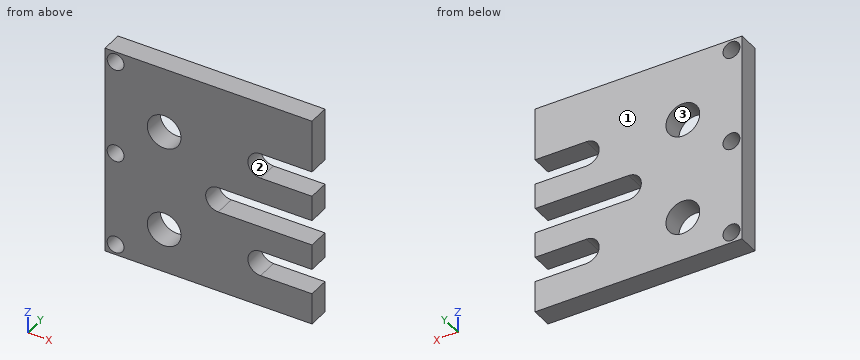
from build123d import *

# Parameters (mm, degrees)
F0_R     = 2
F0_R_2   = 4
F1_DEPTH = 5


with BuildPart() as f1:
    # F0 (on Front) → F1 (new body)
    with BuildSketch(Plane.XZ):
        with BuildLine():
            Line((-9.071991, 28.153977), (-9.071683, 40.657913))
            Line((-9.071683, 40.657913), (-58.072915, 40.657913))
            Line((-58.072915, 40.657913), (-58.072915, -9.342087))
            Line((-58.072915, -9.342087), (-9.072915, -9.342087))
            Line((-9.072915, -9.342087), (-9.072732, -1.896336))
            Line((-9.072732, -1.896336), (-21.245276, -1.896336))
            ThreePointArc((-21.245276, -1.896336), (-24.245276, 1.103664), (-21.245276, 4.103664))
            Line((-21.245276, 4.103664), (-9.082483, 4.103664))
            Line((-9.082483, 4.103664), (-9.072584, 4.103664))
            Line((-9.072584, 4.103664), (-9.072436, 10.135129))
            Line((-9.072436, 10.135129), (-31.243636, 10.135129))
            ThreePointArc((-31.243636, 10.135129), (-34.243636, 13.135129), (-31.243636, 16.135129))
            Line((-31.243636, 16.135129), (-9.072288, 16.135129))
            Line((-9.072288, 16.135129), (-9.07214, 22.145314))
            Line((-9.07214, 22.145314), (-21.245276, 22.145314))
            ThreePointArc((-21.245276, 22.145314), (-24.245275, 25.144246), (-21.24741, 28.145313))
            Line((-21.24741, 28.145313), (-9.071991, 28.153977))
        make_face()
        with Locations((-55.572915, -6.842087)):
            Circle(F0_R, mode=Mode.SUBTRACT)
        with Locations((-44.072376, 1.109681)):
            Circle(F0_R_2, mode=Mode.SUBTRACT)
        with Locations((-55.572915, 15.657913)):
            Circle(F0_R, mode=Mode.SUBTRACT)
        with Locations((-44.072434, 25.151316)):
            Circle(F0_R_2, mode=Mode.SUBTRACT)
        with Locations((-55.572915, 38.157913)):
            Circle(F0_R, mode=Mode.SUBTRACT)
    extrude(amount=F1_DEPTH)


solid = f1.part
Could you check a few things on this model? Use its own coordinates, in mm. Face numbers are marked on the shaded views. Give positions to 0.01 mm unless a question says otherwise; leave off trailing zeros. Loops run counter-clockwise (first coordinate to the right, second up) from the corner with the lowest first, then second, coordinate; pieces in that order, holes last. Notation, with made-up numbers: (61.5, 73.5) -> (72.5, 73.5) arc R5 cw to (72.5, 79.5) -> close; hole circle Ø5 at (58, 83). An arc over 180 degrees is marked (long way). Return JSON: item names as keys, results as strings.
Item 1: If we section it at A-A on x = -28: List the corners of the cut face in (y, z) for me, plus the area to 3 significant figures.
Geometry results:
{"outline": "(-5, -9.34) -> (0, -9.34) -> (0, 10.14) -> (-5, 10.14) -> close; (-5, 16.14) -> (0, 16.14) -> (0, 40.66) -> (-5, 40.66) -> close", "area": "220 mm²"}
Item 2: We'd pull the mould along X, two halves only. Please class the marked faces 1, 2 and 3: +X half, -X half, draft (parallel to the pull), parting line (faces both ways), or undercut.
Geometry results:
{"face 1": "draft", "face 2": "+X half", "face 3": "undercut"}
Item 3: I'm going to push a flat-ended pin straight in: pin 1 (7 mm diameter, centred on x = -44.07, z = 25.15, fed in from -Y). Where does the tip first touch, or does it pass through?
Geometry results:
{"pin 1": "passes through"}
Item 4: If we section it at D-D on x = -14: List the corners of the cut face in (y, z) for me.
Geometry results:
{"outline": "(-5, -9.34) -> (0, -9.34) -> (0, -1.9) -> (-5, -1.9) -> close; (-5, 4.1) -> (0, 4.1) -> (0, 10.14) -> (-5, 10.14) -> close; (-5, 16.14) -> (0, 16.14) -> (0, 22.15) -> (-5, 22.15) -> close; (-5, 28.15) -> (0, 28.15) -> (0, 40.66) -> (-5, 40.66) -> close"}
Item 5: If we section it at C-C on x = -43: List the corners of the cut face in (y, z) for me, plus the area to 3 significant figures.
Geometry results:
{"outline": "(-5, -9.34) -> (0, -9.34) -> (0, -2.74) -> (-5, -2.74) -> close; (-5, 4.96) -> (0, 4.96) -> (0, 21.3) -> (-5, 21.3) -> close; (-5, 29) -> (0, 29) -> (0, 40.66) -> (-5, 40.66) -> close", "area": "173 mm²"}
Item 6: I need wall thicknesses on L1, parallel to Z at x = -55.5, y = -3.75; L2, parallel to Z at x = -17, y = -2.8; L3, parallel to Z at x = -28.5, y = -2.45. Which ranges of each line are inside material? Lowest first, please. Write a range as from..to.
Geometry results:
{"L1": "z = -9.34..-8.84, -4.84..13.66, 17.66..36.16, 40.16..40.66", "L2": "z = -9.34..-1.9, 4.1..10.14, 16.14..22.15, 28.15..40.66", "L3": "z = -9.34..10.14, 16.14..40.66"}
Item 7: If we section it at B-B on z = 15: List the corners of the cut face in (x, y) for me.
Geometry results:
{"outline": "(-58.07, -5) -> (-57.46, -5) -> (-57.46, 0) -> (-58.07, 0) -> close; (-53.68, -5) -> (-33.59, -5) -> (-33.59, 0) -> (-53.68, 0) -> close"}
